from build123d import *

# Parameters (mm, degrees)
EXTRUDE_4_DEPTH     = 8
SKETCH_7_W          = 13
SKETCH_7_H          = 6.499106166
CUT_EXTRUDE_3_DEPTH = 31.054117854
SKETCH_8_R          = 1.6
CUT_EXTRUDE_4_DEPTH = 31.054117854


with BuildPart() as part:
    # 草图6 → 凸台-拉伸4 (new body)
    with BuildSketch(Plane.XY):
        Polygon((-5, 20), (-10.5, 20), (-10.5, 27), (5.5, 27), (5.5, 20), (0, 15.33359454), (0, 0), (-5, 0), align=None)
    extrude(amount=EXTRUDE_4_DEPTH)

    # 草图7 → 切除-拉伸3 (cut, through all)
    with BuildSketch(Plane(origin=(0, 0, 0), x_dir=(-1, 0, 0), z_dir=(0, 0, -1))):
        with Locations((3, 24.249553083)):
            Rectangle(SKETCH_7_W, SKETCH_7_H)
    extrude(amount=-CUT_EXTRUDE_3_DEPTH, mode=Mode.SUBTRACT)

    # 草图8 → 切除-拉伸4 (cut, through all)
    with BuildSketch(Plane(origin=(0, 0, 0), x_dir=(0, 0, -1), z_dir=(1, 0, 0))):
        with Locations((-4, 10)):
            Circle(SKETCH_8_R)
    extrude(amount=-CUT_EXTRUDE_4_DEPTH, mode=Mode.SUBTRACT)


solid = part.part
For this review, take the finished solid that the model builds, in its own axes (mm). A direction names the side the tool comes from. Coordinates: 2 decimals unless noted, no trailing zeros. Loops run counter-clockwise (first coordinate to the right, second up) from the corner with the lowest first, then second, coordinate; pieces in that order, holes last. Notation, with made-up numbers: (49, -1.5) - (69, -1.5) arc R23 ccw to (69, 25.5) - close; hole circle Ø4 at (22.5, 28). An arc over 180 degrees is marked (long way). Use a Markdown table: item, result. Add a question column.
Item 1: Mouldability with a two-part tool opening along X and no side actions: class faces 1 (the face through (-3, 21, 4)), 2 (the face through (-2, 14, 0)), 3 (the face through (0, 8, 4)), 4 (the face through (-5, 10, 2)) as pulls with the +X half, pulls with the -X half, needs draft (parallel to the pull), parting line crosses it, or undercut.
Item 2: We need section C-C (x = -1). Give the boundary of the cut face in (y, z).
Item 3: We need section A-A (y = 10). Give the boundary of the cut face in (x, z).
Item 4: Insertion check: pin 1 Ø2.5 at (x, z) = (-3, 5.5) entering from +Y; pin 2 Ø4 at (y, z) = (7.5, 5.5) entering from -X. Each pin has a flat end and moves straight along its axis. Give the tip position at first contact, or say it passes through.
Item 5: We need section B-B (z = 4). Give the boundary of the cut face in (x, y), and give its area (3 significant figures).
Item 6: For line 1 (Y direction, x = -3.85, z = 4); line 2 (X direction, y = 23.5, z = 1.75); line 3 (X direction, y = 8, z = 2.5), list the stretches that pass through material, from the lowest coordinate up.
Item 7: We need section D-D (z = 7). Give the boundary of the cut face in (x, y).
Item 8: Tool access review of faces 5 (the face through (-8, 20, 4)), 6 (the face through (3.5, 24, 4)), 7 (the face through (-10, 27, 4)): name each direction out of +Z, -Z, +X, -X, +Y, -Y from which nothing blocks a thin tool from reaching the whole face with its end or side.
Results list:
| question | item | result |
|---|---|---|
| 1 | face 1 | undercut |
| 1 | face 2 | needs draft |
| 1 | face 3 | pulls with the +X half |
| 1 | face 4 | pulls with the -X half |
| 2 | outline | (0, 0) - (21, 0) - (21, 8) - (0, 8) - close; hole circle Ø3.2 at (10, 4) |
| 3 | outline | (-5, 0) - (0, 0) - (0, 2.4) - (-5, 2.4) - close; (-5, 5.6) - (0, 5.6) - (0, 8) - (-5, 8) - close |
| 4 | pin 1 | stops at y = 21 |
| 4 | pin 2 | stops at x = -5 |
| 5 | outline | (-10.5, 20) - (-5, 20) - (-5, 11.6) - (0, 11.6) - (0, 15.33) - (5.5, 20) - (5.5, 27) - (3.5, 27) - (3.5, 21) - (-9.5, 21) - (-9.5, 27) - (-10.5, 27) - close; (-5, 0) - (0, 0) - (0, 8.4) - (-5, 8.4) - close |
| 5 | area | 131 mm^2 |
| 6 | line 1 | y = 0 to 8.4, 11.6 to 21 |
| 6 | line 2 | x = -10.5 to -9.5, 3.5 to 5.5 |
| 6 | line 3 | x = -5 to 0 |
| 7 | outline | (-10.5, 20) - (-5, 20) - (-5, 0) - (0, 0) - (0, 15.33) - (5.5, 20) - (5.5, 27) - (3.5, 27) - (3.5, 21) - (-9.5, 21) - (-9.5, 27) - (-10.5, 27) - close |
| 8 | face 5 | +Z, -Z, -X, -Y |
| 8 | face 6 | +Z, -Z, +Y |
| 8 | face 7 | +Z, -Z, +X, -X, +Y |
